from build123d import *

# Parameters (mm, degrees)
F1_DEPTH = 63.5
F0_W     = 25.3345113873
F0_H     = 19.05
F0_H_2   = 7.9502
F0_H_3   = 4.7498
F2_DEPTH = 25.4
F3_DEPTH = 8.255


with BuildPart() as f1:
    # F0 (on Front) → F1 (new body, symmetric)
    with BuildSketch(Plane.XZ):
        Polygon((22.225, 9.525), (-41.275, 9.525), (-41.275, -9.525), (41.275, -9.525), (41.275, 9.525), align=None)
    extrude(amount=F1_DEPTH, both=True)

    # F0 (on Front) → F2 (join, symmetric)
    with BuildSketch(Plane.XZ):
        with BuildLine():
            Line((22.225, 27.0002), (22.225, 9.525))
            Line((22.225, 9.525), (41.275, 9.525))
            Line((41.275, 9.525), (41.275, 27.0002))
            ThreePointArc((41.275, 27.0002), (45.9246798487, 38.2255201513), (57.15, 42.8752))
            Line((57.15, 42.8752), (60.325, 42.8752))
            Line((60.325, 42.8752), (60.325, 61.9252))
            Line((60.325, 61.9252), (57.15, 61.9252))
            add(Edge.make_bspline(
                [(54.7094854303, 61.8398256242), (55.5196441787, 61.8701239826), (56.3331729653, 61.8985622867), (57.15, 61.9252)],
                knots=[109.9108367824, 109.9108367824, 109.9108367824, 109.9108367824, 111.5045361635, 111.5045361635, 111.5045361635, 111.5045361635], degree=3))
            ThreePointArc((54.7094854303, 61.8398256242), (31.6060124849, 50.8174275218), (22.225, 27.0002))
        make_face()
        with Locations((72.9922556937, 52.4002)):
            Rectangle(F0_W, F0_H)
        Polygon((85.6595113873, 66.675), (85.6595113873, 61.9252), (85.6595113873, 42.8752), (85.6595113873, 34.925), (111.125, 34.925), (111.125, 66.675), align=None)
        with Locations((72.9922556937, 38.9001)):
            Rectangle(F0_W, F0_H_2)
        with Locations((72.9922556937, 64.3001)):
            Rectangle(F0_W, F0_H_3)
    extrude(amount=F2_DEPTH, both=True)

    # F0 (on Front) → F3 (join, symmetric)
    with BuildSketch(Plane.XZ):
        with BuildLine():
            add(Edge.make_bspline(
                [(-41.275, 9.525), (-41.0082168827, 48.8137659642), (-1.1638034837, 59.7502735026), (54.7094854303, 61.8398256242)],
                knots=[0, 0, 0, 0, 109.9108367824, 109.9108367824, 109.9108367824, 109.9108367824], degree=3))
            Line((-41.275, 9.525), (22.225, 9.525))
            Line((22.225, 9.525), (22.225, 27.0002))
            ThreePointArc((22.225, 27.0002), (31.6060124849, 50.8174275218), (54.7094854303, 61.8398256242))
        make_face()
    extrude(amount=F3_DEPTH, both=True)

    # F0 (on Front) → F4 (revolve)
    with BuildSketch(Plane.XZ):
        Polygon((85.6595113873, 66.675), (85.6595113873, 61.9252), (85.6595113873, 42.8752), (85.6595113873, 34.925), (111.125, 34.925), (111.125, 66.675), align=None)
    revolve(axis=Axis((111.125, 0, 50.8), (0, 0, -1)))


solid = f1.part
Geometry check sheet. Reference: the model listing, model coordinates, mm. A direction names the side the tool comes from. Round coordinates to 2 decimals unless told otherwise and drop trailing zeros. Write each loop counter-clockwise with the first axis right and the second up, starting at its lowest first coordinate (ties: lowest second). Pieces come first, ordered by that corner, then holes. Notation, with made-up numbers: (-28, 79.5) -> (-11, 79.5) arc R18 cw to (-11, 104.5) -> close; hole circle Ø7 at (55.25, 47.25). An arc over 180 degrees is marked (long way). One line per item, written item: value. Start each with the question number.
(1) Scan lines: line 1 (Z direction, x = 63, y = 24.5) (3 decimals); line 2 (Y direction, x = 98, z = 35); line 3 (Z direction, x = -30.5, y = -15) (3 decimals). Record each from-to range of solid material in increasing order. Write a range as [from, to].
(2) Cross-section at B-B, the plane y = -54. Record the cut outline in (x, z) (3 decimals), and give its area (3 significant figures).
(3) Cross-section at A-A, the plane x = 92. Record the cut outline in (y, z) (3 decimals), and give its area (3 significant figures).
(4) Go/stop test with flat-tipped pins: pin 1 Ø8.5 at (y, z) = (6, 40) entering from -X; pin 2 Ø2.5 at (x, y) = (58.5, 0.5) entering from -Z; pin 3 Ø2 at (x, z) = (11.5, 32.5) entering from -Y (3 decimals); pin 4 Ø17 at (x, z) = (65, 25.5) entering from +Y. Record where each tip stops, or that it passes through.
(5) Access from +Z, -Z, +X, -X, +Y, -Y to the whole of each face (thin tool, end or side, straight path). Record for faces 1 (the flat face through (-3, 8.255, 30)), 2 (the flat face through (-3, -8.255, 30)), 3 (the flat face through (60.325, 0, 64)).
(6) Draft check along X on faces 4 (the flat face through (60.325, 0, 39)), 5 (the flat face through (65, 25.4, 45)), 6 (the flat face through (41.275, -1, 4)). Enter one of: +X half, -X half, draft (parallel to the pull), parting line (faces both ways), or undercut.
Answer:
1. line 1: [34.925, 66.675]
1. line 2: [-25.4, 25.4]
1. line 3: [-9.525, 9.525]
2. outline: (-41.275, -9.525) -> (41.275, -9.525) -> (41.275, 9.525) -> (-41.275, 9.525) -> close
2. area: 1,570 mm²
3. outline: (-25.4, 34.925) -> (25.4, 34.925) -> (25.4, 66.675) -> (-25.4, 66.675) -> close
3. area: 1,610 mm²
4. pin 1: x = -32.69
4. pin 2: z = 42.88
4. pin 3: y = -8.255
4. pin 4: through
5. face 1: +Z, -X, +Y
5. face 2: +Z, -X, -Y
5. face 3: +Z, -X, +Y, -Y
6. face 4: undercut
6. face 5: draft
6. face 6: +X half
